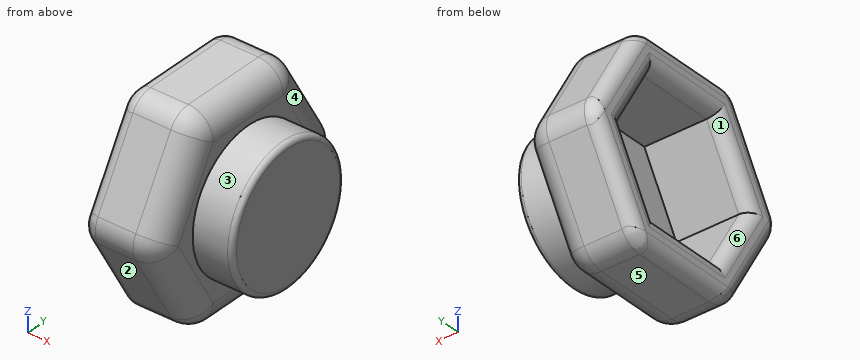
```python
from build123d import *

# Parameters (mm, degrees)
PAD005_DEPTH    = 4.62
POCKET004_DEPTH = 3
FILLET_R        = 0.5
FILLET001_R     = 1
SKETCH011_R     = 2.75
POCKET005_DEPTH = 1.6
FILLET002_R     = 1
FILLET003_R     = 0.2


with BuildPart() as part:
    # Sketch009 → Pad005 (new body)
    with BuildSketch(Plane.YZ):
        Polygon((4.618802, 0), (2.309401, 4), (-2.309401, 4), (-4.618802, 0), (-2.309401, -4), (2.309401, -4), align=None)
    extrude(amount=PAD005_DEPTH)

    # Sketch010 → Pocket004 (cut)
    with BuildSketch(Plane.YZ):
        Polygon((3.175426, 0), (1.587713, 2.75), (-1.587713, 2.75), (-3.175426, 0), (-1.587713, -2.75), (1.587713, -2.75), align=None)
    extrude(amount=POCKET004_DEPTH, mode=Mode.SUBTRACT)

    # Fillet
    fillet_edges = [part.edges().sort_by_distance(p)[0] for p in [
        (0, 3.464102, -2),
        (0, 3.464102, 2),
        (0, 0, 4),
        (0, -3.464102, 2),
        (0, -3.464102, -2),
        (0, 0, -4),
        (0, 2.38157, -1.375),
        (0, 2.38157, 1.375),
        (0, 0, 2.75),
        (0, -2.38157, 1.375),
        (0, -2.38157, -1.375),
        (0, 0, -2.75),
    ]]
    fillet(fillet_edges, radius=FILLET_R)

    # Fillet001
    fillet001_edges = [part.edges().sort_by_distance(p)[0] for p in [
        (2.56, 4.618802, 0),
        (2.56, 2.309401, 4),
        (2.56, -2.309401, 4),
        (2.56, 2.309401, -4),
        (2.56, -2.309401, -4),
        (2.56, -4.618802, 0),
    ]]
    fillet(fillet001_edges, radius=FILLET001_R)

    # Sketch011 (on Face5 of Fillet001) → Pocket005 (cut)
    with BuildSketch(Plane.YZ.offset(4.62)):
        Polygon((4.618802, 0), (2.309401, 4), (-2.309401, 4), (-4.618802, 0), (-2.309401, -4), (2.309401, -4), align=None)
        Circle(SKETCH011_R, mode=Mode.SUBTRACT)
    extrude(amount=-POCKET005_DEPTH, mode=Mode.SUBTRACT)

    # Fillet002
    fillet002_edges = [part.edges().sort_by_distance(p)[0] for p in [
        (3.02, 0, -4),
    ]]
    fillet(fillet002_edges, radius=FILLET002_R)

    # Fillet003
    fillet003_edges = [part.edges().sort_by_distance(p)[0] for p in [
        (4.62, -2.75, 0),
    ]]
    fillet(fillet003_edges, radius=FILLET003_R)


with BuildPart() as part_1:
    # Body001 placement: moved
    add(part.part.moved(Location((22, -6.35, 11.5))))


solid = part_1.part
```
Check sheet for the modelled part. Datum: model origin and axes. Units: mm. Face numbers are marked on the shaded views. A direction names the side the tool comes from. Round coordinates to 2 decimals unless told otherwise and drop trailing zeros. Order: outer loops, then holes, each group sorted by start corner. A loop starts at its lowest first (then second) coordinate and runs counter-clockwise, first axis right, second up. Notation, with made-up numbers: M 13,75.25 L 65,75.25 A19 ccw 65,80.25 Z; hole C -14.75,-33 d10. An arc over 180 degrees is marked long. Answer in a Markdown table with one row per item.
(1) Set-up check for the marked faces 1, 2 and 3: record each of +Z, -Z, +X, -X, +Y, -Y from which the full face is reachable in a straight line by a thin tool's end or side.
Findings:
| item | result |
|---|---|
| face 1 | -X |
| face 2 | -Z, +X, -X, -Y |
| face 3 | +X |
(2) Section check C-C on x = 25.6. Record the boundary of the cut face in (y, z), plus the area to 3 significant figures.
Findings:
| item | result |
|---|---|
| outline | C -6.35,11.5 d5.5 |
| area | 23.8 mm^2 |
(3) Gauge pin test, flat ends, axial feed: pin 1 (1 mm diameter, centred on x = 25, y = -9, fed in from +Z); pin 2 (1.5 mm diameter, centred on x = 26, y = -4.5, fed in from -Z). Record the tip position at first contact, or that the pin passes through.
Findings:
| item | result |
|---|---|
| pin 1 | stops at z = 15.04 |
| pin 2 | stops at z = 8.98 |
(4) Draft check along Z on the marked faces 4, 5 and 6. Enter one of: +Z half, -Z half, draft (parallel to the pull), parting line (faces both ways), or undercut.
Findings:
| item | result |
|---|---|
| face 4 | +Z half |
| face 5 | -Z half |
| face 6 | undercut |
(5) Material ranges on line 1 along Z through (x, y) = (22.65, -7); line 2 along Y through (x, z) = (23.35, 14); line 3 along X through (y, z) = (-7.5, 13), recorded low to high. Write a range as from..to.
Findings:
| item | result |
|---|---|
| line 1 | z = 7.5..8.75, 14.25..15.5 |
| line 2 | y = -9.53..-8.08, -4.62..-3.17 |
| line 3 | x = 25..26.62 |
(6) Section check A-A on x = 22.95. Record the boundary of the cut face in (y, z).
Findings:
| item | result |
|---|---|
| outline | M -10.68,11 L -8.95,8 A1 ccw -8.08,7.5 L -4.62,7.5 A1 ccw -3.75,8 L -2.02,11 A1 ccw -2.02,12 L -3.75,15 A1 ccw -4.62,15.5 L -8.08,15.5 A1 ccw -8.95,15 L -10.68,12 A1 ccw Z; hole M -9.53,11.5 L -7.94,8.75 L -4.76,8.75 L -3.17,11.5 L -4.76,14.25 L -7.94,14.25 Z |
(7) Section check B-B on y = -6.35. Record the boundary of the cut face in (x, z), plus the area to 3 significant figures.
Findings:
| item | result |
|---|---|
| outline | M 22,8 A0.5 ccw 22.5,7.5 L 24.02,7.5 A1 ccw 25.02,8.5 L 25.02,8.75 L 26.42,8.75 A0.2 ccw 26.62,8.95 L 26.62,14.05 A0.2 ccw 26.42,14.25 L 25.02,14.25 L 25.02,14.5 A1 ccw 24.02,15.5 L 22.5,15.5 A0.5 ccw 22,15 L 22,14.75 A0.5 ccw 22.5,14.25 L 25,14.25 L 25,8.75 L 22.5,8.75 A0.5 ccw 22,8.25 Z |
| area | 15.8 mm^2 |
